from build123d import *

# Parameters (mm, degrees)
SKETCH1_W                 = 31.8
SKETCH1_H                 = 15.8
BOSS_EXTRUDE1_DEPTH       = 9.6
SKETCH2_R                 = 2.4
BOSS_EXTRUDE2_DEPTH       = 1.8
SKETCH3_W                 = 29.4
SKETCH3_H                 = 13.4
CUT_EXTRUDE1_DEPTH        = 8.6
SKETCH4_R                 = 1.3
CUT_EXTRUDE2_DEPTH        = 1.7
SKETCH5_R                 = 3.11
SKETCH5_R_2               = 2.4
BOSS_EXTRUDE3_DEPTH       = 8.6
BOSS_EXTRUDE4_DEPTH       = 6.3
SKETCH7_W                 = 0.6
SKETCH7_H                 = 0.2
SKETCH7_W_2               = 0.2
SKETCH7_H_2               = 0.6
BOSS_EXTRUDE5_DEPTH       = 8.6
MIRROR2_COPY_1_SKETCH_W   = 0.6
MIRROR2_COPY_1_SKETCH_H   = 0.2
MIRROR2_COPY_1_SKETCH_W_2 = 0.2
MIRROR2_COPY_1_SKETCH_H_2 = 0.6
MIRROR2_COPY_1_DEPTH      = 8.6


with BuildPart() as part:
    # Sketch1 → Boss-Extrude1 (new body)
    with BuildSketch(Plane(origin=(0, 0, 0), x_dir=(1, 0, 0), z_dir=(0, 1, 0))):
        Rectangle(SKETCH1_W, SKETCH1_H)
    extrude(amount=-BOSS_EXTRUDE1_DEPTH)

    # Sketch2 → Boss-Extrude2 (add)
    with BuildSketch(Plane(origin=(0, 0, 0), x_dir=(1, 0, 0), z_dir=(0, 1, 0))):
        with Locations(Location((-12, 4, 0), (0, 0, 270))):
            Circle(SKETCH2_R)
        with Locations(Location((-4, 4, 0), (0, 0, 270))):
            Circle(SKETCH2_R)
        with Locations(Location((4, 4, 0), (0, 0, 270))):
            Circle(SKETCH2_R)
        with Locations(Location((12, 4, 0), (0, 0, 270))):
            Circle(SKETCH2_R)
        with Locations(Location((12, -4, 0), (0, 0, 270))):
            Circle(SKETCH2_R)
        with Locations(Location((4, -4, 0), (0, 0, 270))):
            Circle(SKETCH2_R)
        with Locations(Location((-4, -4, 0), (0, 0, 270))):
            Circle(SKETCH2_R)
        with Locations(Location((-12, -4, 0), (0, 0, 270))):
            Circle(SKETCH2_R)
    extrude(amount=BOSS_EXTRUDE2_DEPTH)

    # Sketch3 → Cut-Extrude1 (cut)
    with BuildSketch(Plane.XZ.offset(9.6)):
        Rectangle(SKETCH3_W, SKETCH3_H)
    extrude(amount=-CUT_EXTRUDE1_DEPTH, mode=Mode.SUBTRACT)

    # Sketch4 → Cut-Extrude2 (cut)
    with BuildSketch(Plane.XZ.offset(1)):
        with Locations(Location((-12, 4, 0), (0, 0, 270))):
            Circle(SKETCH4_R)
        with Locations(Location((-4, 4, 0), (0, 0, 270))):
            Circle(SKETCH4_R)
        with Locations(Location((4, 4, 0), (0, 0, 270))):
            Circle(SKETCH4_R)
        with Locations(Location((12, 4, 0), (0, 0, 270))):
            Circle(SKETCH4_R)
        with Locations(Location((12, -4, 0), (0, 0, 270))):
            Circle(SKETCH4_R)
        with Locations(Location((4, -4, 0), (0, 0, 270))):
            Circle(SKETCH4_R)
        with Locations(Location((-4, -4, 0), (0, 0, 270))):
            Circle(SKETCH4_R)
        with Locations(Location((-12, -4, 0), (0, 0, 270))):
            Circle(SKETCH4_R)
    extrude(amount=-CUT_EXTRUDE2_DEPTH, mode=Mode.SUBTRACT)

    # Sketch5 → Boss-Extrude3 (add)
    # profile 1 of 3: a face of its own
    with BuildSketch(Plane.XZ.offset(1)):
        with Locations(Location((-8, 0, 0), (0, 0, 90))):
            Circle(SKETCH5_R)
        with Locations(Location((-8, 0, 0), (0, 0, 90))):
            Circle(SKETCH5_R_2, mode=Mode.SUBTRACT)
    # profile 2 of 3: a face of its own
    with BuildSketch(Plane.XZ.offset(1)):
        with Locations(Location((0, 0, 0), (0, 0, 90))):
            Circle(SKETCH5_R)
        with Locations(Location((0, 0, 0), (0, 0, 90))):
            Circle(SKETCH5_R_2, mode=Mode.SUBTRACT)
    # profile 3 of 3: a face of its own
    with BuildSketch(Plane.XZ.offset(1)):
        with Locations(Location((8, 0, 0), (0, 0, 90))):
            Circle(SKETCH5_R)
        with Locations(Location((8, 0, 0), (0, 0, 90))):
            Circle(SKETCH5_R_2, mode=Mode.SUBTRACT)
    extrude(amount=BOSS_EXTRUDE3_DEPTH)

    # Sketch6 → Boss-Extrude4 (add)
    with BuildSketch(Plane.XZ.offset(1)):
        with BuildLine():
            Line((-0.4, 6.7), (-0.4, 3.084169256))
            ThreePointArc((-0.4, 3.084169256), (0, 3.11), (0.4, 3.084169256))
            Line((0.4, 3.084169256), (0.4, 6.7))
            Line((0.4, 6.7), (-0.4, 6.7))
        make_face()
        with BuildLine():
            Line((-0.4, -3.084169256), (-0.4, -6.7))
            Line((-0.4, -6.7), (0.4, -6.7))
            Line((0.4, -6.7), (0.4, -3.084169256))
            ThreePointArc((0.4, -3.084169256), (0, -3.11), (-0.4, -3.084169256))
        make_face()
    extrude(amount=BOSS_EXTRUDE4_DEPTH)

    # Sketch7 → Boss-Extrude5 (add)
    with BuildSketch(Plane.XZ.offset(1)):
        with Locations((-12, 6.6)):
            Rectangle(SKETCH7_W, SKETCH7_H)
        with Locations((-4, 6.6)):
            Rectangle(SKETCH7_W, SKETCH7_H)
        with Locations((-14.6, 4)):
            Rectangle(SKETCH7_W_2, SKETCH7_H_2)
    boss_extrude5 = extrude(amount=BOSS_EXTRUDE5_DEPTH)

    # Mirror1: Boss-Extrude5 across plane
    add(boss_extrude5.mirror(Plane(origin=(0, 0, 0), x_dir=(0, 0, 1), z_dir=(1, 0, 0))))

    # Mirror2: Boss-Extrude5 across plane
    add(boss_extrude5.mirror(Plane.XY))

    # Mirror2 copy 1 sketch → Mirror2 copy 1 (add)
    with BuildSketch(Plane(origin=(0, -1, 0), x_dir=(-1, 0, 0), z_dir=(0, -1, 0))):
        with Locations((-12, 6.6)):
            Rectangle(MIRROR2_COPY_1_SKETCH_W, MIRROR2_COPY_1_SKETCH_H)
        with Locations((-4, 6.6)):
            Rectangle(MIRROR2_COPY_1_SKETCH_W, MIRROR2_COPY_1_SKETCH_H)
        with Locations((-14.6, 4)):
            Rectangle(MIRROR2_COPY_1_SKETCH_W_2, MIRROR2_COPY_1_SKETCH_H_2)
    extrude(amount=MIRROR2_COPY_1_DEPTH)


solid = part.part
Work out the finished part from the listing and answer in its coordinate system (mm). A direction names the side the tool comes from. Coordinates: 2 decimals unless noted, no trailing zeros. Write each loop counter-clockwise with the first axis right and the second up, starting at its lowest first coordinate (ties: lowest second). Pieces come first, ordered by that corner, then holes. Notation, with made-up numbers: M 57.5,71.5 L 101.5,71.5 A27 cw 101.5,93.5 Z; hole C 70.5,-25 d3. An arc over 180 degrees is marked long. Use one line per item in the form item = value. Start each with the question number.
1. Each of these flat-tipped pins is pushed along its axis until it touches: P1, Ø3, axis at x = 0, z = 0, coming from the -Y side; P2, Ø3, axis at x = -1, z = 0.5, coming from the +Y side; P3, Ø6, axis at x = -12, z = 0, coming from the -Y side. Where does it stop, or does it pass through?
2. A tool of negligible diameter and unlimited length cuts with its end or side. For faces 3 (the face through (-12, 1.8, 4)), 4 (the face through (-14, -5, 6.7)), from which of +Z, -Z, +X, -X, +Y, -Y can it reach the whole face along a straight path? Write none if from no direction.
3. The part is cut by section B-B (x = -8). Give the vertices of the cut face in (y, z), plus the area to 3 significant figures.
4. The part is cut by section A-A (y = -8.75). Give the number of separate pieces and of enclosed holes in the cut face, plus the area to 3 significant figures.
5. Straight lines are drawn through the part: probe 1 along X at (y, z) = (-2.25, -5.5); probe 2 along X at (y, z) = (-0.4, -4); probe 3 along Z at (x, y) = (8, -3). For each, find the intervals that lie inside material, in ascending order. Write a range as from..to.
6. The mould has two halves that part along Z. Classify faces 1 (the face through (-6, -9.6, 2)), 2 (the face through (1, -5, 6.7)): released by +Z, released by -Z, zero draft, split by the parting line, or undercut.
Evaluation:
q1.P1 = -1
q1.P2 = 0
q1.P3 = -9.6
q2.face_3 = +Z, -Z, +X, -X, +Y
q2.face_4 = -Y
q3.outline = M -9.6,-7.9 L 0,-7.9 L 0,7.9 L -9.6,7.9 L -9.6,6.7 L -1,6.7 L -1,3.11 L -9.6,3.11 L -9.6,2.4 L -1,2.4 L -1,-2.4 L -9.6,-2.4 L -9.6,-3.11 L -1,-3.11 L -1,-6.7 L -9.6,-6.7 Z
q3.area = 48.7 mm^2
q4.separate_pieces = 4
q4.enclosed_holes = 4
q4.area = 147 mm^2
q5.probe_1 = -15.9..-14.7, -0.4..0.4, 14.7..15.9
q5.probe_2 = -15.9..-13.3, -10.7..-5.3, -2.7..2.7, 5.3..10.7, 13.3..15.9
q5.probe_3 = -7.9..-6.7, -3.11..-2.4, 2.4..3.11, 6.7..7.9
q6.face_1 = zero draft
q6.face_2 = undercut
